```python
from build123d import *

# Parameters (mm, degrees)
CYLINDER005_R     = 8.7
CYLINDER005_DEPTH = 40
CYLINDER003_R     = 8.7
CYLINDER003_DEPTH = 40
CYLINDER007_R     = 10.75
CYLINDER007_DEPTH = 40


with BuildPart() as outletextension:
    # Cylinder005 → Cylinder005 (new body)
    with BuildSketch(Plane(origin=(20, 65.3, 13.5), x_dir=(1, 0, 0), z_dir=(0, -1, 0))):
        Circle(CYLINDER005_R)
    extrude(amount=CYLINDER005_DEPTH)


with BuildPart() as inside:
    # Cylinder003 → Cylinder003 (new body)
    with BuildSketch(Plane(origin=(20, 36.3, 13.5), x_dir=(1, 0, 0), z_dir=(0, -1, 0))):
        Circle(CYLINDER003_R)
    extrude(amount=CYLINDER003_DEPTH)

    # Fusion001: union OutletExtension
    add(outletextension.part)


with BuildPart() as housingoutlet:
    # Cylinder007 → Cylinder007 (new body)
    with BuildSketch(Plane(origin=(20, 59.3, 13.5), x_dir=(1, 0, 0), z_dir=(0, -1, 0))):
        Circle(CYLINDER007_R)
    extrude(amount=CYLINDER007_DEPTH)


with BuildPart() as bloweroutletadapter:
    # Cone001 → Cone001 (revolve)
    with BuildSketch(Plane(origin=(20, 65.3, 13.5), x_dir=(-1, 0, 0), z_dir=(0, 0, 1))):
        Polygon((0, 0), (10.92, 0), (11.19, 21), (0, 21), align=None)
    revolve(axis=Axis((20, 65.3, 13.5), (0, -1, 0)))

    # Fusion: union HousingOutlet
    add(housingoutlet.part)

    # Cut: cut inside
    add(inside.part, mode=Mode.SUBTRACT)


solid = bloweroutletadapter.part
```
The model under review builds one solid part; all positions refer to its coordinate system, in mm. A direction names the side the tool comes from. Round coordinates to 2 decimals unless told otherwise and drop trailing zeros. Order: outer loops, then holes, each group sorted by start corner. A loop starts at its lowest first (then second) coordinate and runs counter-clockwise, first axis right, second up. Notation, with made-up numbers: (-25, -38) -> (19, -38) arc R25 ccw to (19, -6) -> close; hole circle Ø2 at (-7, 4). An arc over 180 degrees is marked (long way). Use a Markdown table: item, result.
Q1. For line 1 (Z direction, x = 20, y = 43.5); line 2 (X direction, y = 32.5, z = 13.5); line 3 (Y direction, x = 26, z = 4.5), list the stretches that pass through material, from the lowest coordinate up.
Values:
| item | result |
|---|---|
| line 1 | z = 2.75 to 4.8, 22.2 to 24.25 |
| line 2 | x = 9.25 to 11.3, 28.7 to 30.75 |
| line 3 | y = 44.3 to 65.3 |
Q2. Mouldability with a two-part tool opening along X and no side actions: class faces 1 (the conical face through (22.397, 54.653, 24.294)), 2 (the flat face through (30, 44.3, 9)), 3 (the cylindrical face through (18.867, 42.622, 22.126)) as +X half, -X half, draft (parallel to the pull), parting line (faces both ways), or undercut.
Values:
| item | result |
|---|---|
| face 1 | parting line |
| face 2 | draft |
| face 3 | undercut |
Q3. We need section B-B on y = 52. Write out the cut boundary in (x, z).
Values:
| item | result |
|---|---|
| outline | circle Ø22.18 at (20, 13.5); hole circle Ø17.4 at (20, 13.5) |
Q4. Clearance check with flat-ended pins moving along their axes: P1, Ø10, axis at x = 19, z = 12, coming from the +Y side; P2, Ø1.5, axis at y = 26.5, z = 9.5, coming from the +X side; P3, Ø5, axis at x = 16, y = 42, coming from the -Z side; P4, Ø1.5, axis at y = 25.5, z = 18.5, coming from the -X side. State where each tip first meets the part, or that it passes through.
Values:
| item | result |
|---|---|
| P1 | passes through |
| P2 | stops at x = 30.25 |
| P3 | stops at z = 2.73 |
| P4 | stops at x = 10.13 |
Q5. We need section A-A on y = 33. Write out the cut boundary in (x, z).
Values:
| item | result |
|---|---|
| outline | circle Ø21.5 at (20, 13.5); hole circle Ø17.4 at (20, 13.5) |
Q6. Tool access review of faces 4 (the cylindrical face through (18.6, 31.98, 24.16)), 5 (the flat face through (29, 19.3, 14)): name each direction out of +Z, -Z, +X, -X, +Y, -Y from which nothing blocks a thin tool from reaching the whole face with its end or side.
Values:
| item | result |
|---|---|
| face 4 | -Y |
| face 5 | +Z, -Z, +X, -X, -Y |
